from build123d import *

# Parameters (mm, degrees)
BOSS_EXTRUDE1_DEPTH    = 28.575
F_6_32_TAPPED_HOLE1_D  = 2.7051
F_6_CLEARANCE_HOLE1_D  = 3.7973
CUT_EXTRUDE1_START     = -3.175
CUT_EXTRUDE1_OUTLINE_R = 1.35255
CUT_EXTRUDE1_DEPTH     = 3.175
SKETCH9_W              = 12.7
SKETCH9_H              = 22.225
CUT_EXTRUDE2_DEPTH     = 45.22263278
FILLET1_R              = 3.175


# Read off the part's stored shape, not the designer's step: Cut-Extrude1
with BuildPart() as part:
    # Sketch1 → Boss-Extrude1 (new body)
    with BuildSketch(Plane.XY):
        Polygon((0, -25.4), (0, 0), (-25.4, 0), (-25.4, -3.175), (-3.175, -3.175), (-3.175, -25.4), align=None)
    extrude(amount=BOSS_EXTRUDE1_DEPTH)

    # 6-32 Tapped Hole1 (through all)
    with Locations(Plane(origin=(-8.255, 0, 3.175), x_dir=(1, 0, 0), z_dir=(0, 1, 0))):
        with Locations((0, 0), (-10.3, -22.2)):
            Hole(F_6_32_TAPPED_HOLE1_D / 2)

    # 6 Clearance Hole1 (through all)
    with Locations(Plane(origin=(-3.175, -12.7, 12.7), x_dir=(0, -1, 0), z_dir=(-1, 0, 0))):
        with Locations((0, 0), (6.35, -9.525)):
            Hole(F_6_CLEARANCE_HOLE1_D / 2)

    # Cut-Extrude1 outline → Cut-Extrude1 (cut)
    with BuildSketch(Plane(origin=(0, 0, 0), x_dir=(1, 0, 0), z_dir=(0, 1, 0)).offset(CUT_EXTRUDE1_START)):
        with BuildLine():
            ThreePointArc((-23.161554656, -24.551311816), (-21.241762382, -25.769160339), (-19.223133004, -26.815053658))
            ThreePointArc((-19.223133004, -26.815053658), (-17.114946342, -26.043133004), (-17.886866996, -23.934946342))
            ThreePointArc((-17.886866996, -23.934946342), (-19.659563377, -23.016475956), (-21.345464145, -21.946999958))
            ThreePointArc((-21.345464145, -21.946999958), (-23.555665329, -22.341110632), (-23.161554656, -24.551311816))
        make_face()
        with Locations((-18.555, -25.375)):
            Circle(CUT_EXTRUDE1_OUTLINE_R, mode=Mode.SUBTRACT)
    extrude(amount=CUT_EXTRUDE1_DEPTH, mode=Mode.SUBTRACT)

    # Sketch9 → Cut-Extrude2 (cut, through all)
    with BuildSketch(Plane.ZY.offset(3.175)):
        with Locations((22.225, -14.2875)):
            Rectangle(SKETCH9_W, SKETCH9_H)
    extrude(amount=-CUT_EXTRUDE2_DEPTH, mode=Mode.SUBTRACT)

    # Fillet1
    fillet1_edges = [part.edges().sort_by_distance(p)[0] for p in [
        (-3.175, -3.175, 7.9375),
        (-1.5875, -3.175, 15.875),
    ]]
    fillet(fillet1_edges, radius=FILLET1_R)


solid = part.part
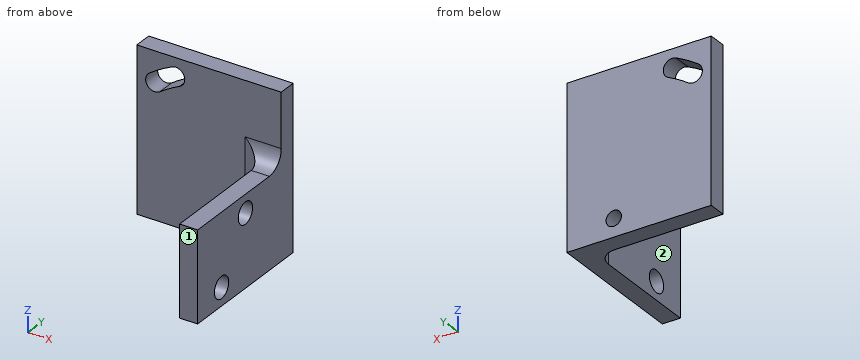
Verification items for the finished model (mm, model axes). Face numbers are marked on the shaded views. A direction names the side the tool comes from. Coordinates: 2 decimals unless noted, no trailing zeros. Write each loop counter-clockwise with the first axis right and the second up, starting at its lowest first coordinate (ties: lowest second). Pieces come first, ordered by that corner, then holes. Notation, with made-up numbers: (-14.5, 4.5) -> (-0.5, 4.5) arc R31 ccw to (-0.5, 30.5) -> close; hole circle Ø4 at (80.5, 2.5). An arc over 180 degrees is marked (long way). One line per item, written item: value. Start each with the question number.
Q1. Cross-section at C-C on x = -8. Enter the section's corners in (y, z) (3 decimals), and give its area (3 significant figures).
Q2. Go/stop test with flat-tipped pins: P1, Ø2.5, axis at x = -1.5, y = -14.5, coming from the +Z side (3 decimals); P2, Ø4, axis at x = -19, z = 8, coming from the +Y side; P3, Ø5, axis at y = -20.5, z = 5, coming from the -X side (3 decimals); P4, Ø12, axis at x = -21, z = 12, coming from the -Y side (3 decimals). Record where each tip stops, or that it passes through.
Q3. Access from +Z, -Z, +X, -X, +Y, -Y to the whole of each face (thin tool, end or side, straight path). Record for the marked faces 1 and 2.
Q4. Cross-section at A-A on z = 12.7. Enter the section's corners in (x, y) (3 decimals).
Q5. Cross-section at B-B on y = -19.05. Enter the section's corners in (x, z) (3 decimals).
Q6. Thickness scan on L1, parallel to Z at x = -0.65, y = -12.7 (3 decimals); L2, parallel to Z at x = -2.35, y = -19.05 (3 decimals); L3, parallel to Y at x = -19.5, z = 14.75 (3 decimals). Record the ranges inside material, lowest first. Write a range as from..to.
Q7. Cross-section at D-D on z = 9.25. Enter the section's corners in (x, y) (3 decimals).
Checked values:
1. outline: (-3.175, 0) -> (0, 0) -> (0, 1.847) -> (-3.175, 1.847) -> close; (-3.175, 4.503) -> (0, 4.503) -> (0, 28.575) -> (-3.175, 28.575) -> close
1. area: 82.3 mm²
2. P1: stops at z = 15.875
2. P2: stops at y = 0
2. P3: stops at x = -3.175
2. P4: stops at y = -3.175
3. face 1: +Z, -Z, +X, -X, -Y
3. face 2: +Z, -Z, -X, -Y
4. outline: (-25.4, -3.175) -> (-6.35, -3.175) arc R3.175 cw to (-3.175, -6.35) -> (-3.175, -10.801) -> (0, -10.801) -> (0, 0) -> (-25.4, 0) -> close; (-3.175, -25.4) -> (0, -25.4) -> (0, -14.599) -> (-3.175, -14.599) -> close
5. outline: (-3.175, 0) -> (0, 0) -> (0, 1.276) -> (-3.175, 1.276) -> close; (-3.175, 5.074) -> (0, 5.074) -> (0, 15.875) -> (-3.175, 15.875) -> close
6. L1: z = 0..10.801, 14.599..15.875
6. L2: z = 0..1.276, 5.074..15.875
6. L3: y = -3.175..0
7. outline: (-25.4, -3.175) -> (-6.35, -3.175) arc R3.175 cw to (-3.175, -6.35) -> (-3.175, -25.4) -> (0, -25.4) -> (0, 0) -> (-25.4, 0) -> close
